```python
from build123d import *

# Parameters (mm, degrees)
F0_R     = 175
F1_DEPTH = 8
F2_R     = 175
F2_R_2   = 170
F3_DEPTH = 260
F4_R     = 80
F5_DEPTH = 100
F6_W     = 6
F6_H     = 15
F7_DEPTH = 185
F8_R     = 170
F9_DEPTH = 100


with BuildPart() as f1:
    # F0 (on Top) → F1 (new body)
    with BuildSketch(Plane.XY):
        Circle(F0_R)
    extrude(amount=F1_DEPTH)

    # F2 (on face) → F3 (join)
    with BuildSketch(Plane.XY.offset(8)):
        Circle(F2_R)
        Circle(F2_R_2, mode=Mode.SUBTRACT)
    extrude(amount=F3_DEPTH)

    # F4 (on face) → F5 (join)
    with BuildSketch(Plane.XY.offset(8)):
        Circle(F4_R)
    extrude(amount=F5_DEPTH)

    # F6 (on Front) → F7 (join, symmetric)
    with BuildSketch(Plane.XZ):
        Polygon((-54, 220), (0, 220), (0, 228), (-60, 228), (-60, 220), align=None)
        Polygon((0, 228), (0, 220), (54, 220), (60, 220), (60, 228), align=None)
        with Locations((-57, 212.5)):
            Rectangle(F6_W, F6_H)
        with Locations((57, 212.5)):
            Rectangle(F6_W, F6_H)
    extrude(amount=F7_DEPTH, both=True)

    # F8 (on face) → F9 (cut)
    with BuildSketch(Plane.XY.offset(268)):
        Circle(F8_R)
    extrude(amount=-F9_DEPTH, mode=Mode.SUBTRACT)


solid = f1.part
```
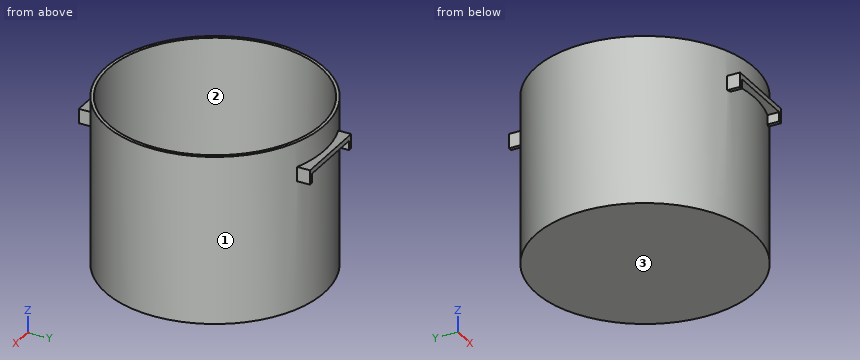
Model file for the job. Use its own axes, mm. Face numbers are marked on the shaded views. Coordinates: 2 decimals unless noted, no trailing zeros. Order: outer loops, then holes, each group sorted by start corner. A loop starts at its lowest first (then second) coordinate and runs counter-clockwise, first axis right, second up. Notation, with made-up numbers: M 87.25,-9.5 L 133.25,-9.5 A28 cw 133.25,23.5 Z; hole C 26.5,2.5 d6. An arc over 180 degrees is marked long. Answer as CSV lines item,"result".
(1) Band-saw the part on D-D, the plane y = 147.5. List the corners of the cut face in (x, z), then the cut area to 3 significant figures.
Geometry says:
outline,"M -94.17,0 L 94.17,0 L 94.17,268 L 84.52,268 L 84.52,8 L -84.52,8 L -84.52,268 L -94.17,268 Z"
area,"6,530 mm2"
(2) Band-saw the part on A-A, the plane x = 0. List the corners of the cut face in (y, z).
Geometry says:
outline,"M -185,220 L -175,220 L -175,0 L 175,0 L 175,220 L 185,220 L 185,228 L 175,228 L 175,268 L 170,268 L 170,8 L 80,8 L 80,108 L -80,108 L -80,8 L -170,8 L -170,268 L -175,268 L -175,228 L -185,228 Z"
(3) Band-saw the part on B-B, the plane z = 38. List the corners of the cut face in (x, y), then the cut area to 3 significant figures.
Geometry says:
outline,"C 0,0 d350; C 0,0 d160; hole C 0,0 d340"
area,"25,500 mm2"
(4) Wall check: line 1 along Y through (x, z) = (0, 98); line 2 along Y through (x, z) = (0, 141); line 3 along X through (y, z) = (-49, 21). Give the ranges that are in metal, low to high.
Geometry says:
line 1,"y = -175 to -170, -80 to 80, 170 to 175"
line 2,"y = -175 to -170, 170 to 175"
line 3,"x = -168 to -162.79, -63.24 to 63.24, 162.79 to 168"
(5) Pull direction Y, two halves, no side cores. Call the marked faces 1, 2 and 3: +Y half, -Y half, draft (parallel to the pull), parting line (faces both ways), or undercut.
Geometry says:
face 1,"parting line"
face 2,"undercut"
face 3,"draft"
(6) Flat gauge pins, fed straight in: pin 1 (3 mm diameter, centred on x = 56.5, y = -174, fed in from -Z); pin 2 (1.5 mm diameter, centred on y = 147.5, z = 62, fed in from +X); pin 3 (7.5 mm diameter, centred on y = -172.5, z = 215, fed in from +X). Where does each tip first touch, or does it go through?
Geometry says:
pin 1,"stops at z = 205"
pin 2,"stops at x = 95.34"
pin 3,"stops at x = 60"
(7) Band-saw the part on C-C, the plane y = 0. List the corners of the cut face in (x, z), then the cut area to 3 significant figures.
Geometry says:
outline,"M -175,0 L 175,0 L 175,268 L 170,268 L 170,8 L 80,8 L 80,108 L -80,108 L -80,8 L -170,8 L -170,268 L -175,268 Z"
area,"21,400 mm2"
